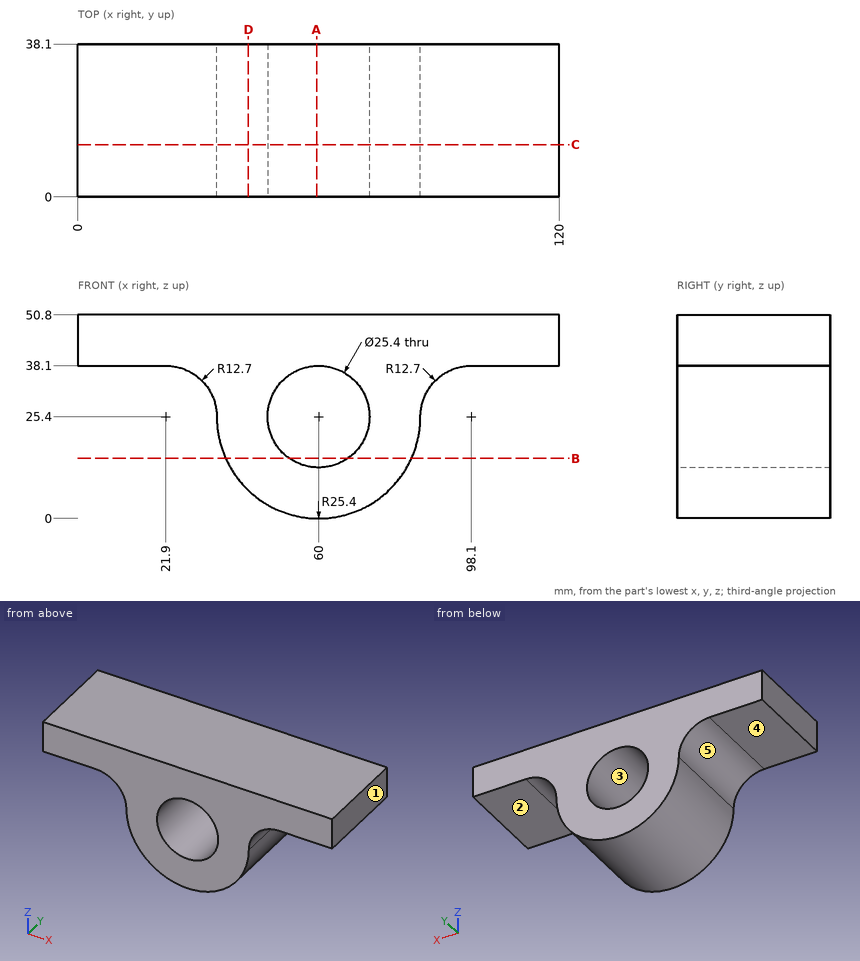
Here's the drawing with two shaded views (mm, measured from the low corner). I have some questions. A direction names the side the tool comes from. Round coordinates to 2 decimals unless told otherwise and drop trailing zeros. Loops run counter-clockwise (first coordinate to the right, second up) from the corner with the lowest first, then second, coordinate; pieces in that order, holes last.
Item 1: If we mould it in two halves opening along X, with no side actions, what happens to the marked faces 3, 4 and 5? For each: +X half, -X half, draft (parallel to the pull), parting line (faces both ways), or undercut.
Item 2: Will these pins go through, and if not, where does the flat tip stop? pin 1 Ø1 at (x, y) = (17.5, 9) entering from -Z; pin 2 Ø10 at (x, y) = (78, 17) entering from -Z; pin 3 Ø1 at (x, z) = (50, 5.5) entering from -Y; pin 4 Ø3 at (y, z) = (17, 33) entering from +X.
Item 3: Suppose I cut it at D-D, the plane x = 42.5. Write out the boundary of the cut face in (y, z), then the cut area to 3 significant figures.
Item 4: Suppose I cut it at C-C, the plane y = 13. Write out the boundary of the cut face in (x, z), then the cut area to 3 significant figures.
Item 5: Which directions (+Z, -Z, +X, -X, +Y, -Y) give clear straight access to the entire face, cutting with the end or side of a thin tool? Please do the marked faces 1 and 2.
Item 6: Please list where these lines run through material, in increasing order: L1, parallel to Z at x = 60, y = 12; L2, parallel to X at y = 15, z = 25; L3, parallel to Z at x = 8.5, y = 17.
Item 7: Suppose I cut it at B-B, the plane z = 15. Write out the boundary of the cut face in (x, y).
Item 8: Suppose I cut it at A-A, the plane x = 59.5. Write out the boundary of the cut face in (y, z).
Reported:
1. face 3: undercut
1. face 4: draft
1. face 5: -X half
2. pin 1: stops at z = 38.1
2. pin 2: stops at z = 3.58
2. pin 3: stops at y = 0
2. pin 4: stops at x = 89.24
3. outline: (0, 6.99) - (38.1, 6.99) - (38.1, 50.8) - (0, 50.8) - close
3. area: 1,670 mm2
4. outline: (0, 38.1) - (21.9, 38.1) arc R12.7 cw to (34.6, 25.4) arc R25.4 ccw to (85.4, 25.4) arc R12.7 cw to (98.1, 38.1) - (120, 38.1) - (120, 50.8) - (0, 50.8) - close; hole circle Ø25.4 at (60, 25.4)
4. area: 2,750 mm2
5. face 1: +Z, -Z, +X, +Y, -Y
5. face 2: -Z, +X, +Y, -Y
6. L1: z = 0 to 12.7, 38.1 to 50.8
6. L2: x = 34.6 to 47.31, 72.69 to 85.4
6. L3: z = 38.1 to 50.8
7. outline: (36.83, 0) - (52.71, 0) - (52.71, 38.1) - (36.83, 38.1) - close; (67.29, 0) - (83.17, 0) - (83.17, 38.1) - (67.29, 38.1) - close
8. outline: (0, 0) - (38.1, 0) - (38.1, 12.71) - (0, 12.71) - close; (0, 38.09) - (38.1, 38.09) - (38.1, 50.8) - (0, 50.8) - close
